Study the drawing (mm; zero at the part's minimum x, y, z) and answer. A direction names the side the tool comes from. Round coordinates to 2 decimals unless told otherwise and drop trailing zeros. Write each loop counter-clockwise with the first axis right and the second up, starting at its lowest first coordinate (ties: lowest second). Pieces come first, ordered by that corner, then holes.
(1) A cutting plane is placed at B-B, the plane y = 3. Give the vertices of the cut face in (x, z), and give its area (3 significant figures).
(2) A cutting plane is placed at D-D, the plane x = 1.75. Give the vertices of the cut face in (y, z), and give its area (3 significant figures).
(3) The mould has two halves that part along X. Classify the marked faces 1, 2 and 3: +X half, -X half, draft (parallel to the pull), parting line (faces both ways), or undercut.
(4) A cutting plane is placed at A-A, the plane x = 5. Give the vertices of the cut face in (y, z).
(5) Find the intervals of material crossed by probe 1 along Y at (x, z) = (5, 3.25); probe 2 along Z at (x, y) = (1.25, 4.5); probe 3 along Y at (x, z) = (3.75, 1.8), in increasing order.
(6) For the marked faces 4 and 5, determine the directions among +Z, -Z, +X, -X, +Y, -Y from which every point of the face is accessible in a straight line to the end or side of a thin tool.
(7) Each of these flat-tipped pins is pushed along its axis until it touches: pin 1 Ø1.5 at (x, z) = (2.5, 3) entering from -Y; pin 2 Ø4 at (x, y) = (5, 15) entering from -Z. Where does it stop, or does it pass through?
(8) A cutting plane is placed at C-C, the plane z = 3.85. Give the vertices of the cut face in (x, y).
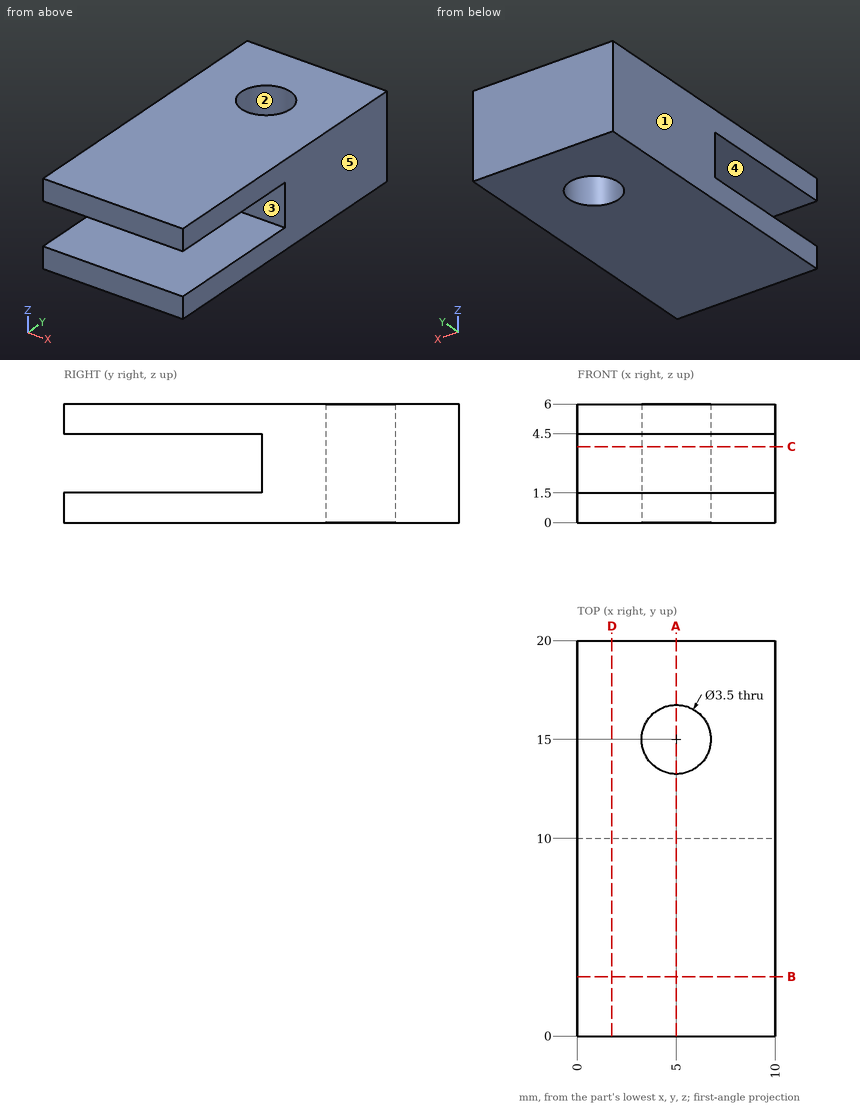
Solutions:
1. outline: (0, 0) - (10, 0) - (10, 1.5) - (0, 1.5) - close; (0, 4.5) - (10, 4.5) - (10, 6) - (0, 6) - close
1. area: 30.0 mm2
2. outline: (0, 0) - (20, 0) - (20, 6) - (0, 6) - (0, 4.5) - (10, 4.5) - (10, 1.5) - (0, 1.5) - close
2. area: 90.0 mm2
3. face 1: -X half
3. face 2: undercut
3. face 3: draft
4. outline: (0, 0) - (13.25, 0) - (13.25, 6) - (0, 6) - (0, 4.5) - (10, 4.5) - (10, 1.5) - (0, 1.5) - close; (16.75, 0) - (20, 0) - (20, 6) - (16.75, 6) - close
5. probe 1: y = 10 to 13.25, 16.75 to 20
5. probe 2: z = 0 to 1.5, 4.5 to 6
5. probe 3: y = 10 to 13.78, 16.22 to 20
6. face 4: +X, -X, -Y
6. face 5: +Z, -Z, +X, +Y, -Y
7. pin 1: stops at y = 10
7. pin 2: stops at z = 0
8. outline: (0, 10) - (10, 10) - (10, 20) - (0, 20) - close; hole circle Ø3.5 at (5, 15)
